```python
from build123d import *

# Parameters (mm, degrees)
SKETCH_1_W          = 68
SKETCH_1_H          = 40
EXTRUDE_1_DEPTH     = 19
SKETCH_2_W          = 44
SKETCH_2_H          = 20
EXTRUDE_2_DEPTH     = 6
SKETCH_4_W          = 2
SKETCH_4_H          = 20
CUT_EXTRUDE_1_DEPTH = 2
SKETCH_5_W          = 68
SKETCH_5_H          = 8
EXTRUDE_3_DEPTH     = 2
MM_1_AT_2_COUNT     = 2
MM_1_AT_2_PITCH     = 15
MM_1_AT_3_COUNT     = 2
MM_1_AT_3_PITCH     = 19.209372712
MM_1_AT_4_COUNT     = 2
MM_1_AT_4_PITCH     = 12
MM_2_D              = 4
MM_2_DEPTH          = 10
MM_2_TIP            = 1.201721238
MM_3_D              = 5
MM_3_DEPTH          = 5
MM_3_TIP            = 1.502151548


with BuildPart() as part:
    # 草图1 → 凸台-拉伸1 (new body)
    with BuildSketch(Plane(origin=(0, 0, 0), x_dir=(1, 0, 0), z_dir=(0, 1, 0))):
        Rectangle(SKETCH_1_W, SKETCH_1_H)
    extrude(amount=EXTRUDE_1_DEPTH)

    # 草图2 → 凸台-拉伸2 (add)
    with BuildSketch(Plane(origin=(0, 19, 0), x_dir=(1, 0, 0), z_dir=(0, 1, 0))):
        Rectangle(SKETCH_2_W, SKETCH_2_H)
    extrude(amount=EXTRUDE_2_DEPTH)

    # 草图4 → 切除-拉伸1 (cut)
    with BuildSketch(Plane(origin=(0, 25, 0), x_dir=(1, 0, 0), z_dir=(0, 1, 0))):
        Rectangle(SKETCH_4_W, SKETCH_4_H)
    extrude(amount=-CUT_EXTRUDE_1_DEPTH, mode=Mode.SUBTRACT)

    # 草图5 → 凸台-拉伸3 (add)
    with BuildSketch(Plane(origin=(0, 19, 0), x_dir=(1, 0, 0), z_dir=(0, 1, 0))):
        Rectangle(SKETCH_5_W, SKETCH_5_H)
    extrude(amount=EXTRUDE_3_DEPTH)

    # 草图7 → 大小mm 暗销孔1 (revolve, cut)
    with BuildSketch(Plane(origin=(17.5, 25, -7.5), x_dir=(0, 0, 1), z_dir=(1, 0, 0))):
        Polygon((0, 0), (0, 4.901290929), (1.5, 4), (1.5, 0), align=None)
    mm_1 = revolve(axis=Axis((17.5, 31.35, -7.5), (0, -1, 0)), mode=Mode.SUBTRACT)

    # 大小mm 暗销孔1 at 2: 大小mm 暗销孔1 ×2
    with Locations(*[(0, 0, i * MM_1_AT_2_PITCH) for i in range(1, MM_1_AT_2_COUNT)]):
        add(mm_1, mode=Mode.SUBTRACT)

    # 大小mm 暗销孔1 at 3: 大小mm 暗销孔1 ×2
    with Locations(*[Vector(-0.6246950475544242, 0, 0.7808688094430305) * (i * MM_1_AT_3_PITCH) for i in range(1, MM_1_AT_3_COUNT)]):
        add(mm_1, mode=Mode.SUBTRACT)

    # 大小mm 暗销孔1 at 4: 大小mm 暗销孔1 ×2
    with Locations(*[(-i * MM_1_AT_4_PITCH, 0, 0) for i in range(1, MM_1_AT_4_COUNT)]):
        add(mm_1, mode=Mode.SUBTRACT)

    # 镜向1: 大小mm 暗销孔1 across plane
    add(mm_1.mirror(Plane(origin=(0, 0, 0), x_dir=(0, 0, 1), z_dir=(1, 0, 0))), mode=Mode.SUBTRACT)

    # 镜向1 copy 1 sketch → 镜向1 copy 1 (revolve, cut)
    with BuildSketch(Plane(origin=(-17.5, 25, 7.5), x_dir=(0, 0, 1), z_dir=(-1, 0, 0))):
        Polygon((0, 0), (0, -4.901290929), (1.5, -4), (1.5, 0), align=None)
    revolve(axis=Axis((-17.5, 31.35, 7.5), (0, 1, 0)), mode=Mode.SUBTRACT)

    # 镜向1 copy 2 sketch → 镜向1 copy 2 (revolve, cut)
    with BuildSketch(Plane(origin=(-5.5, 25, 7.5), x_dir=(0, 0, 1), z_dir=(-1, 0, 0))):
        Polygon((0, 0), (0, -4.901290929), (1.5, -4), (1.5, 0), align=None)
    revolve(axis=Axis((-5.5, 31.35, 7.5), (0, 1, 0)), mode=Mode.SUBTRACT)

    # 镜向1 copy 3 sketch → 镜向1 copy 3 (revolve, cut)
    with BuildSketch(Plane(origin=(-5.5, 25, -7.5), x_dir=(0, 0, 1), z_dir=(-1, 0, 0))):
        Polygon((0, 0), (0, -4.901290929), (1.5, -4), (1.5, 0), align=None)
    revolve(axis=Axis((-5.5, 31.35, -7.5), (0, 1, 0)), mode=Mode.SUBTRACT)

    # 大小mm 暗销孔2
    with Locations(Plane(origin=(21, 0, 0), x_dir=(0, 0, -1), z_dir=(0, -1, 0))):
        with Locations((0, 0), (0, -42)):
            Hole(MM_2_D / 2, depth=MM_2_DEPTH)
            with Locations((0, 0, -(MM_2_DEPTH + MM_2_TIP / 2))):  # 118° drill point
                Cone(0, MM_2_D / 2, MM_2_TIP, mode=Mode.SUBTRACT)

    # 大小mm 暗销孔3
    with Locations(Plane(origin=(34, 7.7, -10), x_dir=(0, 0, 1), z_dir=(1, 0, 0))):
        with Locations((0, 0), (20, 0)):
            Hole(MM_3_D / 2, depth=MM_3_DEPTH)
            with Locations((0, 0, -(MM_3_DEPTH + MM_3_TIP / 2))):  # 118° drill point
                Cone(0, MM_3_D / 2, MM_3_TIP, mode=Mode.SUBTRACT)


solid = part.part
```
Could you check a few things on this model? Use its own coordinates, in mm. A direction names the side the tool comes from. Coordinates: 2 decimals unless noted, no trailing zeros. Loops run counter-clockwise (first coordinate to the right, second up) from the corner with the lowest first, then second, coordinate; pieces in that order, holes last. Notation, with made-up numbers: M 10,19.5 L 15,19.5 A10 ccw 15,38.5 Z; hole C 85,46 d9. An arc over 180 degrees is marked long. Put each result on its own line as item: value. Start each with the question number.
(1) Will these pins go through, and if not, where does the flat tip stop? P1, Ø6, axis at x = 18.5, z = 8, coming from the +Y side; P2, Ø2.5, axis at x = -17.5, z = -7.5, coming from the +Y side; P3, Ø2, axis at x = 26, z = 12.5, coming from the +Y side; P4, Ø3, axis at x = 0.5, y = 21, coming from the +Z side.
(2) Suppose I cut it at C-C on z = 15. Please give me the cut outline in (x, y), then the cut area to 3 significant figures.
(3) Suppose I cut it at A-A on z = -5. Please give me the cut outline in (x, y), then the cut area to 3 significant figures.
(4) Suppose I cut it at B-B on x = -28.5. Please give me the cut outline in (y, z).
(5) For faces 4 (the face through (28, 21, 0)), 5 (the face through (1, 24, 0)), 6 (the face through (16.49, 23.03, -8.61)), 7 (the face through (-19, 5, 0)), which set-ups out of +Z, -Z, +X, -X, +Y, -Y let a thin tool reach every point of the face, with its end or its side?
(6) Thinking about a two-plate mould opening in X: for faces 1 (the face through (34, 10, 0)), 2 (the face through (28, 20, 4)), 3 (the face through (-21.31, 10.99, -0.16)), which applies, pulls with the +X half, pulls with the -X half, needs draft (parallel to the pull), parting line crosses it, or undercut?
(7) I need wall thicknesses on line 1 (X direction, y = 3.75, z = 0); line 2 (X direction, y = 23.15, z = -7.5); line 3 (X direction, y = 22.3, z = 7.5). Which ranges of each line are inside material? Lowest first, please. Write a range as from..to.
Solutions:
1. P1: stops at y = 25
1. P2: stops at y = 20.85
1. P3: stops at y = 19
1. P4: stops at z = 10
2. outline: M -34,0 L 34,0 L 34,19 L -34,19 Z
2. area: 1,290 mm2
3. outline: M -34,0 L 34,0 L 34,19 L 22,19 L 22,25 L 1,25 L 1,23 L -1,23 L -1,25 L -22,25 L -22,19 L -34,19 Z
3. area: 1,550 mm2
4. outline: M 0,-20 L 19,-20 L 19,-4 L 21,-4 L 21,4 L 19,4 L 19,20 L 0,20 Z
5. face 4: +Z, -Z, +X, +Y
5. face 5: +Z, -Z, +Y
5. face 6: +Y
5. face 7: -Y
6. face 1: pulls with the +X half
6. face 2: needs draft
6. face 3: undercut
7. line 1: x = -34..-23, -19..19, 23..34
7. line 2: x = -22..-19, -16..-7, -4..-1, 1..4, 7..16, 19..22
7. line 3: x = -22..-19, -16..-7, -4..4, 7..16, 19..22
